Build history of the part. All positions in model axes, mm. A direction names the side the tool comes from. Round coordinates to 2 decimals unless told otherwise and drop trailing zeros. Put each result on its own line as item: value. Start each with the question number.
from build123d import *

# Parameters (mm, degrees)
BOSS_EXTRUDE1_DEPTH = 2
SKETCH2_R           = 0.6
CUT_EXTRUDE1_DEPTH  = 2
BOUNDARY_CUT1_START = 0.5
BOUNDARY_CUT1_DEPTH = 1


# Read off the part's stored shape, not the designer's step: Boundary-Cut1
with BuildPart() as part:
    # Sketch1 → Boss-Extrude1 (new body)
    with BuildSketch(Plane.XY):
        with BuildLine():
            ThreePointArc((1.526225881, 1.443320919), (0.844261398, -0.518019494), (2.515834251, -1.75))
            Line((2.515834251, -1.75), (6.849532383, -1.75))
            ThreePointArc((6.849532383, -1.75), (8.181942233, -1.134541314), (8.577159836, 0.278932579))
            add(Edge.make_bspline(
                [(8.577159836, 0.278932579), (8.110700048, 2.179296341), (7.304925461, 2.614034863)],
                knots=[0, 0, 0, 1, 1, 1], degree=2))
            add(Edge.make_bspline(
                [(7.304925461, 2.614034863), (7.441478628, 2.291307156), (7.423521915, 1.987733608), (7.251055322, 1.703314219)],
                knots=[0, 0, 0, 0, 0.668538786, 0.668538786, 0.668538786, 0.668538786], degree=3))
            ThreePointArc((7.251055322, 1.703314219), (6.514478451, 1.717625938), (5.837281377, 1.427532101))
            add(Edge.make_bspline(
                [(5.837281377, 1.427532101), (5.390462193, 2.403045527), (4.664925461, 2.614034863)],
                knots=[0.307788008, 0.307788008, 0.307788008, 1, 1, 1], degree=2))
            add(Edge.make_bspline(
                [(4.664925461, 2.614034863), (4.824318966, 2.283493667), (4.768740332, 1.996314703), (4.498189559, 1.752497972)],
                knots=[0, 0, 0, 0, 0.792020938, 0.792020938, 0.792020938, 0.792020938], degree=3))
            Line((4.498189559, 1.752497972), (4.341055322, 1.703314219))
            ThreePointArc((4.341055322, 1.703314219), (3.775786335, 1.742322367), (3.227683317, 1.598677862))
            ThreePointArc((3.227683317, 1.598677862), (3.156194107, 1.628631099), (3.083448661, 1.655389344))
            add(Edge.make_bspline(
                [(3.083448661, 1.655389344), (2.661448554, 2.428931092), (2.024925461, 2.614034863)],
                knots=[0.392713148, 0.392713148, 0.392713148, 1, 1, 1], degree=2))
            add(Edge.make_bspline(
                [(2.024925461, 2.614034863), (2.317287968, 1.973197345), (1.646435899, 1.518764796)],
                knots=[0, 0, 0, 0.922107406, 0.922107406, 0.922107406], degree=2))
            add(Edge.make_bspline(
                [(1.646435899, 1.518764796), (1.589767438, 1.480377803), (1.526225881, 1.443320919)],
                knots=[0.922107406, 0.922107406, 0.922107406, 1, 1, 1], degree=2))
        make_face()
    extrude(amount=BOSS_EXTRUDE1_DEPTH)

    # Sketch2 → Cut-Extrude1 (cut)
    with BuildSketch(Plane.XY.offset(2)):
        with Locations((6.849532383, 0)):
            Circle(SKETCH2_R)
        with Locations((2.515834251, 0)):
            Circle(SKETCH2_R)
    extrude(amount=-CUT_EXTRUDE1_DEPTH, mode=Mode.SUBTRACT)

    # Boundary-Cut1 outline → Boundary-Cut1 (cut)
    with BuildSketch(Plane.XY.offset(BOUNDARY_CUT1_START)):
        with BuildLine():
            add(Edge.make_bspline(
                [(3.182683317, -1.75), (3.219559269, -1.676248097), (3.293311172, -1.528744291), (3.403939026, -1.307488582), (3.51456688, -1.086232874), (3.588340093, -0.938686449), (3.678709694, -0.757947245), (3.783775446, -0.543015437), (3.935584986, -0.217797229), (4.081534514, 0.110092623), (4.174899608, 0.330404865), (4.258110172, 0.531765281), (4.388021164, 0.690444526), (4.682683317, 0.779920411), (4.97734547, 0.690444526), (5.107256462, 0.531765281), (5.190467027, 0.330404865), (5.28383212, 0.110092623), (5.429781648, -0.217797229), (5.581591188, -0.543015437), (5.686671615, -0.757976596), (5.7401719, -0.864977165)],
                knots=[0, 0, 0, 0, 0.049050349, 0.098100699, 0.147151048, 0.196201398, 0.196201398, 0.267425193, 0.338648988, 0.409872783, 0.481096578, 0.481096578, 0.539598638, 0.598100699, 0.656602759, 0.71510482, 0.71510482, 0.786328615, 0.85755241, 0.928776205, 1, 1, 1, 1], degree=3))
            Line((3.182683317, -1.75), (6.182683317, -1.75))
            Line((6.182683317, -1.75), (5.7401719, -0.864977165))
        make_face()
    extrude(amount=BOUNDARY_CUT1_DEPTH, mode=Mode.SUBTRACT)


solid = part.part
1) Slice it at A-A, the plane y = 0.5. State how many separate pieces and enclosed holes the cut face has, and give its area (3 significant figures).
2) Which spindle directions (+Z, -Z, +X, -X, +Y, -Y) get a long thin tool onto all of the face, cutting with end or side? Do faces 4 (the face through (5, -1, 0.5)), 5 (the face through (0.835, -0.488, 0.986)). Say none if no direction does.
3) Pull direction Y, two halves, no side cores. Call faces 1 (the face through (3.784, 1.743, 0.986)), 2 (the face through (1.916, 0.026, 1.014)), 3 (the face through (5, -1, 1.5)): pulls with the +Y half, pulls with the -Y half, needs draft (parallel to the pull), parting line crosses it, or undercut.
4) Drill centre lines: line 1 (Z direction, x = 4.75, y = -0.95); line 2 (X direction, y = -0.2, z = 0.7); line 3 (X direction, y = 1.85, z = 1.75). Where is each one in solid material? Low to high. Write a range as [from, to].
Taken from the geometry:
1. separate pieces: 3
1. enclosed holes: 1
1. area: 11.8 mm2
2. face 4: -Y
2. face 5: +Z, -Z, -X
3. face 1: pulls with the +Y half
3. face 2: undercut
3. face 3: needs draft
4. line 1: z = [0, 0.5], [1.5, 2]
4. line 2: x = [0.78, 1.95], [3.08, 3.94], [5.42, 6.28], [7.42, 8.59]
4. line 3: x = [1.99, 2.97], [4.59, 5.61], [7.33, 8.01]
